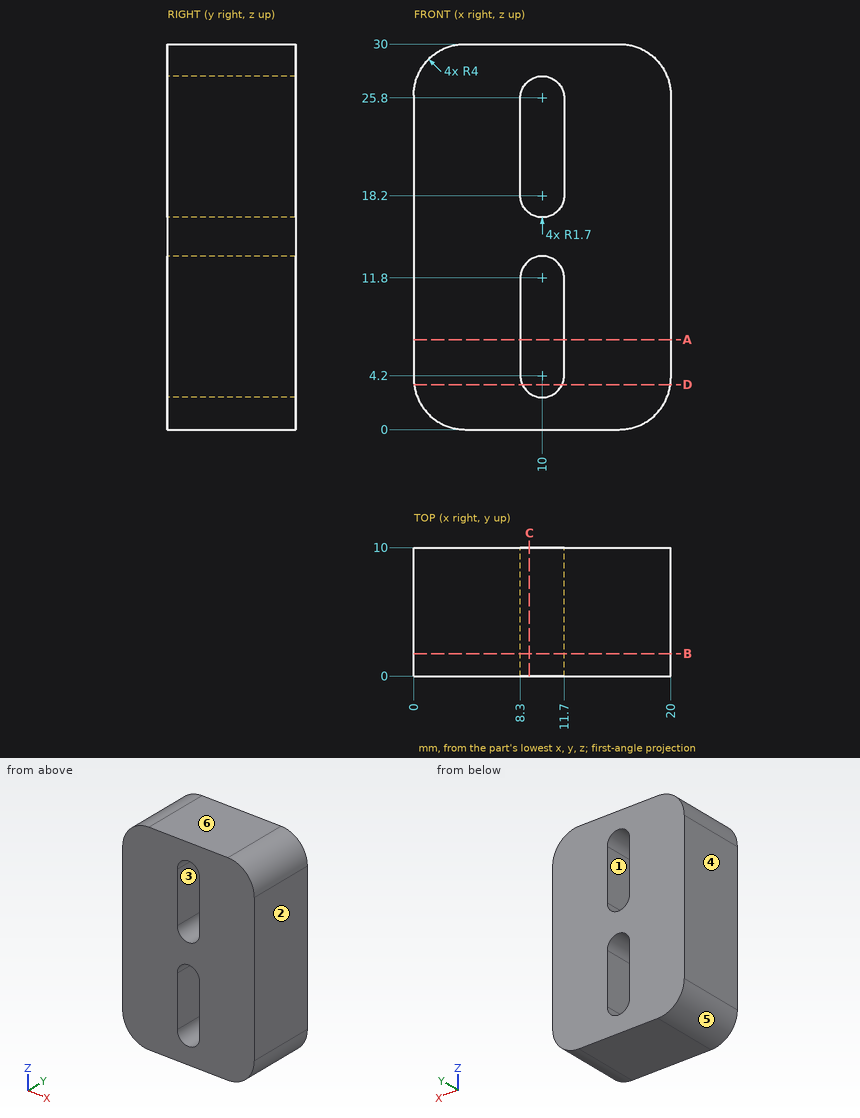
Could you check a few things on this drawing? It's one solid part, dimensions in mm from its lowest x, y, z. A direction names the side the tool comes from. Coordinates: 2 decimals unless noted, no trailing zeros. Write each loop counter-clockwise with the first axis right and the second up, starting at its lowest first coordinate (ties: lowest second). Pieces come first, ordered by that corner, then holes. Notation, with made-up numbers: M 54,-4.75 L 112,-4.75 A31 cw 112,31.25 Z; hole C 81,30.5 d1. An arc over 180 degrees is marked long. Answer as CSV lines item,"result". Start each with the question number.
Q1. For the marked faces 1 and 2, which set-ups out of +Z, -Z, +X, -X, +Y, -Y let a thin tool reach every point of the face, with its end or its side?
Q2. Suppose I cut it at C-C, the plane x = 9. List the corners of the cut face in (y, z) for me.
Q3. Suppose I cut it at D-D, the plane z = 3.5. List the corners of the cut face in (x, y) for me, then the cut area to 3 significant figures.
Q4. Will this pin go through, and if not, where does the flat tip stop? pin 1 Ø10 at (x, z) = (7.5, 18.5) entering from -Y.
Q5. If we mould it in two halves opening along Z, with no side actions, what happens to the marked faces 3, 4, 5 and 6? For each: pulls with the +Z half, pulls with the -Z half, needs draft (parallel to the pull), parting line crosses it, or undercut.
Q6. I need wall thicknesses on probe 1 along X at (y, z) = (8, 23.5); probe 2 along X at (y, z) = (6.75, 26.75); probe 3 along Z at (x, y) = (9, 2). Which ranges of each line are inside material? Lowest first, please. Write a range as [from, to].
Q7. Suppose I cut it at A-A, the plane z = 7. List the corners of the cut face in (x, y) for me.
Q8. Suppose I cut it at B-B, the plane y = 1.75. List the corners of the cut face in (x, z) for me, then the cut area to 3 significant figures.
Entries:
1,face 1,"+Y, -Y"
1,face 2,"+Z, -Z, +X, +Y, -Y"
2,outline,"M 0,0 L 10,0 L 10,2.83 L 0,2.83 Z; M 0,13.17 L 10,13.17 L 10,16.83 L 0,16.83 Z; M 0,27.17 L 10,27.17 L 10,30 L 0,30 Z"
3,outline,"M 0.03,0 L 8.45,0 L 8.45,10 L 0.03,10 Z; M 11.55,0 L 19.97,0 L 19.97,10 L 11.55,10 Z"
3,area,"168 mm²"
4,pin 1,"stops at y = 0"
5,face 3,"undercut"
5,face 4,"needs draft"
5,face 5,"pulls with the -Z half"
5,face 6,"pulls with the +Z half"
6,probe 1,"x = [0, 8.3], [11.7, 20]"
6,probe 2,"x = [0.07, 8.59], [11.41, 19.93]"
6,probe 3,"z = [0, 2.83], [13.17, 16.83], [27.17, 30]"
7,outline,"M 0,0 L 8.3,0 L 8.3,10 L 0,10 Z; M 11.7,0 L 20,0 L 20,10 L 11.7,10 Z"
8,outline,"M 0,4 A4 ccw 4,0 L 16,0 A4 ccw 20,4 L 20,26 A4 ccw 16,30 L 4,30 A4 ccw 0,26 Z; hole M 8.3,4.2 A1.7 ccw 11.7,4.2 L 11.7,11.8 A1.7 ccw 8.3,11.8 Z; hole M 8.3,18.2 A1.7 ccw 11.7,18.2 L 11.7,25.8 A1.7 ccw 8.3,25.8 Z"
8,area,"516 mm²"
